Autodesk Inventor part; units mm, degrees
ref_plane "Work Plane1" through (0, 0, 0) normal (0, -0.7071068, 0.7071068) x (1, 0, 0)
ref_plane "YZ Plane" through (0, 0, 0) normal (1, 0, 0) x (0, 1, 0)
ref_plane "XZ Plane" through (0, 0, 0) normal (0, 1, 0) x (-1, 0, 0)
ref_plane "Work Plane1" through (0, 0, 0) normal (0, -0.7071068, 0.7071068) x (1, 0, 0)
sketch "Sketch1" plane through (0, 0, 0) normal (0, -0.7071068, 0.7071068) x (1, 0, 0)
  circle A0 centre (0, 0) radius 100 construction
  dimension "d1" = 200
sketch "Sketch2" plane through (0, 0, 0) normal (0, 0, 1) x (1, 0, 0)
  line L0 (0, 0) -> (0, 100) construction
  line L1 (0, 0) -> (135.52, 0) construction
  circle A0 centre (0, 74.9294) radius 25 construction
  circle A1 centre (0, 74.9294) radius 12.5 construction
  line L2 (89.6381, 86.81) -> (-89.6381, 86.81) construction
  line L3 (-67.2707, 86.81) -> (-67.2707, 75) construction
  line L4 (-65.5817, 87.4347) -> (-65.5817, 74.9294) construction
  line L5 (65.5817, 87.4347) -> (65.5817, 74.9294) construction
  ellipse E0 centre (0, 0) end of major axis (135.4472, 0) minor radius 99.9294 (65.5817, 87.4347) -> (-65.5817, 87.4347) ccw construction
  line L6 (-62.6083, 85.4701) -> (-62.6083, 74.9294) construction
  line L7 (62.5858, 74.9294) -> (62.5858, 85.4128) construction
  line L8 (-57.1593, 87.4294) -> (-57.1593, 74.9294)
  line L9 (57.1593, 87.4294) -> (-57.1593, 87.4294) construction
  line L10 (57.1593, 87.4294) -> (57.1593, 74.9294)
  line L11 (57.1593, 74.9294) -> (-57.1593, 74.9294)
  spline S0 degree 5 poles (57.1593, 87.4294) (46.1717, 91.2827) (34.8288, 94.1238) (23.2875, 95.9996) (0, 97.8773) (-23.2875, 95.9996) (-34.8288, 94.1238) (-46.1717, 91.2827) (-57.1593, 87.4294) knots 0 0 0 0 0 0 0.5 0.5 0.5 1 1 1 1 1 1
  dimension "d40" = 135.4471
  dimension "d41" = 99.9294
  dimension "d24" = 50
  dimension "d25" = 0
  dimension "d26" = 25
  dimension "d42" = 86.81
  dimension "d43" = 2.9958
  dimension "d44" = 8.4224
  dimension "d45" = 65.5817
  dimension "d46" = 128.19
  dimension "d47" = 132.8524
  dimension "d48" = 0
  dimension "d49" = 65.5817
  dimension "d50" = 69.9383
  dimension "d51" = 24.0564
  dimension "d52" = 74.9294
  dimension "d53" = 85.4129
  dimension "d54" = 74.9294
  dimension "d55" = 100
  dimension "d56" = 85.4701
  dimension "d57" = 74.9294
  dimension "d58" = 75
  dimension "d59" = 155.2197
revolve "Revolution3" add sketch "Sketch2" angle 360 about axis through (57.1593, 74.9294, 0) along (-1, 0, 0)
sketch "Sketch6" plane through (-57.1593, 74.9294, 0) normal (-1, 0, 0) x (0, 0, 1)
  circle A0 centre (0, 0) radius 12.5
  circle A1 centre (0, 0) radius 11
  point P0 (0, -74.9294)
  point P1 (0, 12.5)
  dimension "d61" = 22
extrude "Extrusion3" cut sketch "Sketch6" against normal blind 6 contours A1
sketch "Sketch7" plane through (57.1593, 74.9294, 0) normal (1, 0, 0) x (0, 0, -1)
  circle A0 centre (0, 0) radius 12.5
  circle A1 centre (0, 0) radius 11
  point P0 (0, -74.9294)
  point P1 (0, 12.5)
  dimension "d64" = 22
extrude "Extrusion4" cut sketch "Sketch7" against normal blind 6 contours A1
hole "Hole2" at (57.1593, 74.9294, 0) direction (-1, 0, 0) diameter 8 end through all
properties part number "RollerRedesign5"
The listing builds one solid part. Answer for the finished solid, in the listing's coordinates (mm). A direction names the side the tool comes from. Give positions to 0.01 mm unless a question says otherwise; leave off trailing zeros.
Item 1: For a pull along Y with two mould halves and no side action, classify faces 4 (the face through (-57.159, 80, 10)), 5 (the face through (-54.201, 84.205, 5.914)), 6 (the face through (51.159, 75, -5)) as pulls with the +Y half, pulls with the -Y half, needs draft (parallel to the pull), parting line crosses it, or undercut.
From the geometry:
face 4: needs draft
face 5: undercut
face 6: undercut
Item 2: Given pin 1 Ø6 at (x, y) = (14.5, 85) entering from +Z; pin 2 Ø20 at (y, z) = (74.93, 0) entering from -X; pin 3 Ø5 at (x, z) = (40.5, -3.5) entering from -Y, each flat-ended and moving along its own axis, determine where each tip first touches the part or whether it passes through.
From the geometry:
pin 1: stops at z = 20.25
pin 2: stops at x = -51.16
pin 3: stops at y = 57.22
Item 3: Find the intervals of material crossed by probe 1 along Y at (x, z) = (53, 0); probe 2 along X at (y, z) = (68.5, -3); probe 3 along Y at (x, z) = (-17, -1), in increasing order.
From the geometry:
probe 1: y = 61.03 to 63.93, 85.93 to 88.82
probe 2: x = -51.16 to 51.16
probe 3: y = 53.75 to 71.06, 78.8 to 96.11
Item 4: Which of the six approach directions +Z, -Z, +X, -X, +Y, -Y give full straight-line access (tool end or side, diameter ignored) to faces 1 (the face through (54.201, 84.205, -5.914)), 2 (the face through (57.159, 80, 10)), 3 (the face through (-51.159, 75, 5))?
From the geometry:
face 1: +X
face 2: +Z, -Z, +X, +Y, -Y
face 3: -X
